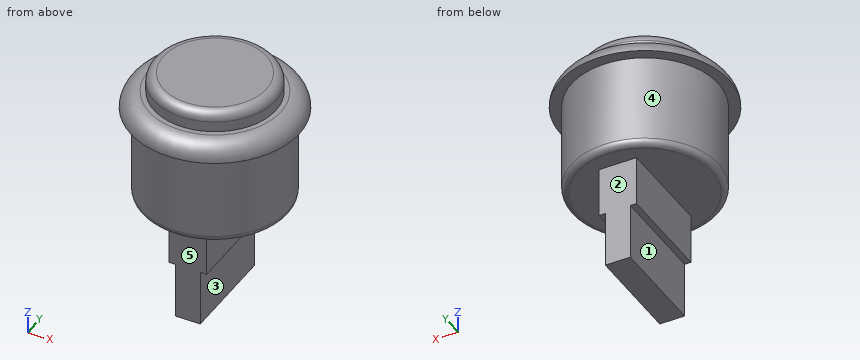
Autodesk Inventor part; units mm, degrees
ref_plane "YZ Plane" through (0, 0, 0) normal (1, 0, 0) x (0, 1, 0)
ref_plane "XZ Plane" through (0, 0, 0) normal (0, 1, 0) x (-1, 0, 0)
ref_plane "XY Plane" through (0, 0, 0) normal (0, 0, 1) x (1, 0, 0)
sketch "Sketch1" plane through (0, 0, 0) normal (0, 0, 1) x (1, 0, 0)
  circle A0 centre (0, 0) radius 11.75
  dimension "d0" = 23.5
extrude "Extrusion1" add sketch "Sketch1" against normal blind 15
sketch "Sketch2" plane through (0, 0, 0) normal (0, 0, 1) x (1, 0, 0)
  circle A0 centre (0, 0) radius 11.75
  circle A1 centre (0, 0) radius 13.5
  dimension "d3" = 27
extrude "Extrusion2" add sketch "Sketch2" along normal blind 2.8 contours A0 | A1
sketch "Sketch3" plane through (0, 0, 2.8) normal (0, 0, 1) x (1, 0, 0)
  circle A0 centre (0, 0) radius 13.5
  circle A1 centre (0, 0) radius 9.75
  dimension "d8" = 19.5
extrude "Extrusion3" add sketch "Sketch3" along normal blind 3.2 contours A1
fillet "Fillet1" radius 1.5 1 edges at (-9.75, 0, 6)
fillet "Fillet2" radius 2.95 1 edges at (-13.5, 0, 2.8)
fillet "Fillet3" radius 1 1 edges at (-11.75, 0, -15)
sketch "Sketch4" plane through (0, 0, -15) normal (0, 0, -1) x (-1, 0, 0)
  circle A0 centre (0, 0) radius 10.75
  line L0 (-3, 8) -> (3, 8)
  line L1 (3, 8) -> (3, -8)
  line L2 (3, -8) -> (-3, -8)
  line L3 (-3, -8) -> (-3, 8)
  point P0 (3, 0)
  point P1 (0, 8)
  dimension "d14" = 6
  dimension "d16" = 16
extrude "Extrusion4" add sketch "Sketch4" along normal blind 8 contours L0 L1 L2 L3
sketch "Sketch5" plane through (0, 0, -23) normal (0, 0, -1) x (-1, 0, 0)
  line L0 (3, 8) -> (-3, 8)
  line L1 (3, -8) -> (3, 8)
  line L2 (-2, 8) -> (2, 8)
  line L3 (2, 8) -> (2, -8)
  line L4 (2, -8) -> (-2, -8)
  line L5 (-2, -8) -> (-2, 8)
  point P0 (0, 0)
  point P1 (2, 0)
  point P2 (3, 0)
  point P3 (0, 8)
  point P4 (0, 8)
  dimension "d19" = 4
  dimension "d21" = 16
extrude "Extrusion5" add sketch "Sketch5" along normal blind 9
properties part number "OBSF-24_button" material "Nylon 6"
Can you work these out from the model? Positions are in its coordinate system, mm. Face numbers are marked on the shaded views. A direction names the side the tool comes from. Give positions to 0.01 mm unless a question says otherwise; leave off trailing zeros. Order: outer loops, then holes, each group sorted by start corner. A loop starts at its lowest first (then second) coordinate and runs counter-clockwise, first axis right, second up. Notation, with made-up numbers: M 33.5,4 L 69.5,4 A28 cw 69.5,26 Z; hole C 70.5,72.5 d5. An arc over 180 degrees is marked long. One line per item, written item: value.
1) I want a section at D-D, the plane z = -16.5. List the corners of the cut face in (x, y) for me, plus the area to 3 significant figures.
Answer sheet:
outline: M -3,-8 L 3,-8 L 3,8 L -3,8 Z
area: 96.0 mm^2
2) On a 3-axis mill with a long thin cutter (end or side, diameter ignored), from which of +Z, -Z, +X, -X, +Y, -Y can I reach the whole of each face in a straight line? I mean the marked faces 1, 2, 3, 4 and 5. Say none if no direction works.
Answer sheet:
face 1: -Z, -X, +Y, -Y
face 2: -Z, +X, -X, +Y
face 3: -Z, +X, +Y, -Y
face 4: -Z
face 5: -Z, +X, -X, -Y
3) For P1, Ø10, axis at y = -5, z = -16.5, coming from the +X side; P2, Ø2.5, axis at y = -0.5, z = -19.5, coming from the +X side; P3, Ø4.5, axis at y = 0, z = -26.5, coming from the -X side, each with a flat end and sliding along its axis, tell me the tip position at first contact or that it passes through.
Answer sheet:
P1: stops at x = 11.73
P2: stops at x = 3
P3: stops at x = -2
4) I want a section at A-A, the plane y = 0. List the corners of the cut face in (x, z) for me.
Answer sheet:
outline: M -13.5,0 L -11.75,0 L -11.75,-14 A1 ccw -10.75,-15 L -3,-15 L -3,-23 L -2,-23 L -2,-32 L 2,-32 L 2,-23 L 3,-23 L 3,-15 L 10.75,-15 A1 ccw 11.75,-14 L 11.75,0 L 13.5,0 A2.95 ccw 10.55,2.8 L 9.75,2.8 L 9.75,4.5 A1.5 ccw 8.25,6 L -8.25,6 A1.5 ccw -9.75,4.5 L -9.75,2.8 L -10.55,2.8 A2.95 ccw Z
5) I want a section at C-C, the plane z = -28. List the corners of the cut face in (x, y) for me, plus the area to 3 significant figures.
Answer sheet:
outline: M -2,-8 L 2,-8 L 2,8 L -2,8 Z
area: 64.0 mm^2
6) I want a section at B-B, the plane x = 0. List the corners of the cut face in (y, z) for me.
Answer sheet:
outline: M -13.5,0 L -11.75,0 L -11.75,-14 A1 ccw -10.75,-15 L -8,-15 L -8,-32 L 8,-32 L 8,-15 L 10.75,-15 A1 ccw 11.75,-14 L 11.75,0 L 13.5,0 A2.95 ccw 10.55,2.8 L 9.75,2.8 L 9.75,4.5 A1.5 ccw 8.25,6 L -8.25,6 A1.5 ccw -9.75,4.5 L -9.75,2.8 L -10.55,2.8 A2.95 ccw Z
7) Please list where these lines run through material, in increasing order: line 1 along Z through (x, y) = (-3.25, -6.75); line 2 along Z through (x, y) = (-2.25, -10.5); line 3 along X through (y, z) = (5.25, -15.5).
Answer sheet:
line 1: z = -15 to 6
line 2: z = -15 to 2.79
line 3: x = -3 to 3
